CAD build for the part. Positions are in the model's coordinates, mm. Face numbers are marked on the shaded views. Coordinates: 2 decimals unless noted, no trailing zeros. Order: outer loops, then holes, each group sorted by start corner. A loop starts at its lowest first (then second) coordinate and runs counter-clockwise, first axis right, second up. Notation, with made-up numbers: M 68,30 L 75,30 A24 ccw 75,68 Z; hole C 42.25,59.25 d3. An arc over 180 degrees is marked long. One line per item, written item: value.
from build123d import *


with BuildPart() as f1:
    # F0 (on Front) → F1 (revolve)
    with BuildSketch(Plane.XZ):
        with BuildLine():
            Line((46, 35), (11, 35))
            Line((11, 35), (11, 19))
            Line((11, 19), (20, 19))
            Line((20, 19), (20, 0))
            Line((20, 0), (0, 0))
            Line((0, 0), (0, -25))
            ThreePointArc((0, -25), (29.515258, -29.454987), (56.400715, -42.42301))
            Line((56.400715, -42.42301), (70.823725, -28))
            Line((70.823725, -28), (70.823725, -22))
            ThreePointArc((70.823725, -22), (61.572329, -16.216507), (51.851852, -11.261768))
            ThreePointArc((51.851852, -11.261768), (47.589249, -7.571892), (46, -2.162709))
            Line((46, -2.162709), (46, 35))
        make_face()
    revolve(axis=Axis((0, 0, 17.5), (0, 0, -1)))


solid = f1.part
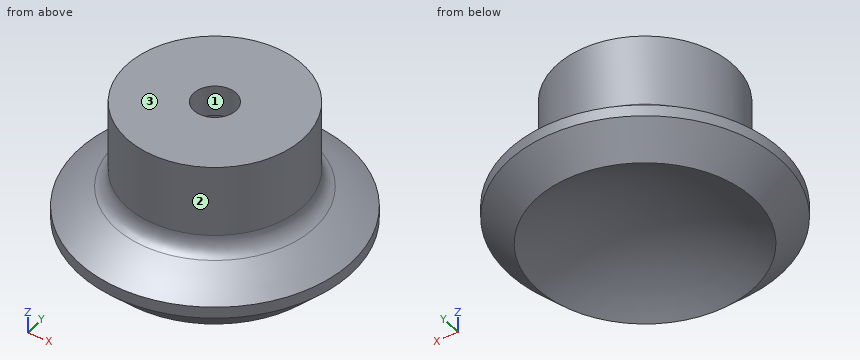
Q1. Mould opens along X. For the marked faces 1, 2 and 3 say: released by +X, released by -X, zero draft, split by the parting line, or undercut.
Recorded:
face 1: undercut
face 2: split by the parting line
face 3: zero draft
Q2. Slice it at A-A (z = 8.5). List the corners of the cut face in (x, y), plus the area to 3 significant figures.
Recorded:
outline: C 0,0 d92; hole C 0,0 d40
area: 5,390 mm^2
Q3. Slice it at B-B (z = -6). List the corners of the cut face in (x, y), plus the area to 3 significant figures.
Recorded:
outline: C 0,0 d93.53
area: 6,870 mm^2
Q4. Drill centre lines: line 1 along X through (y, z) = (0, 9); line 2 along X through (y, z) = (0, 27). Where is each one in solid material? Low to high.
Recorded:
line 1: x = -46 to -20, 20 to 46
line 2: x = -46 to -11, 11 to 46
Q5. Pin check, flat tips, straight feed: pin 1 Ø4 at (y, z) = (-31, 5) entering from +X; pin 2 Ø1 at (x, z) = (-14.5, 9) entering from -Y; pin 3 Ø20 at (x, y) = (0, 0) entering from +Z. Stop position of each tip, or through.
Recorded:
pin 1: stops at x = 35.71
pin 2: stops at y = -43.82
pin 3: stops at z = 0
